from build123d import *

# Parameters (mm, degrees)
SKETCH002_W   = 115
SKETCH002_H   = 101.6
SKETCH002_R   = 3.25
SKETCH002_R_2 = 19.05
SKETCH002_R_3 = 2.1
PAD002_DEPTH  = 6.35
FILLET_R      = 2
SKETCH004_R   = 1.25
SKETCH004_R_2 = 2.75
POCKET_DEPTH  = 6.351


with BuildPart() as part:
    # Sketch002 → Pad002 (new body)
    with BuildSketch(Plane.XZ):
        Rectangle(SKETCH002_W, SKETCH002_H)
        with Locations((19.4, 38.1)):
            Circle(SKETCH002_R, mode=Mode.SUBTRACT)
        with Locations((44.8, 38.1)):
            Circle(SKETCH002_R, mode=Mode.SUBTRACT)
        with Locations((19.4, 12.7)):
            Circle(SKETCH002_R, mode=Mode.SUBTRACT)
        with Locations((44.8, 12.7)):
            Circle(SKETCH002_R, mode=Mode.SUBTRACT)
        with Locations((19.4, -12.7)):
            Circle(SKETCH002_R, mode=Mode.SUBTRACT)
        with Locations((44.8, -12.7)):
            Circle(SKETCH002_R, mode=Mode.SUBTRACT)
        with Locations((19.4, -38.1)):
            Circle(SKETCH002_R, mode=Mode.SUBTRACT)
        with Locations((44.8, -38.1)):
            Circle(SKETCH002_R, mode=Mode.SUBTRACT)
        with Locations((-23.3, -15.1)):
            Circle(SKETCH002_R_2, mode=Mode.SUBTRACT)
        with Locations((-46.85, 8.45)):
            Circle(SKETCH002_R_3, mode=Mode.SUBTRACT)
        with Locations((0.25, 8.45)):
            Circle(SKETCH002_R_3, mode=Mode.SUBTRACT)
        with Locations((-46.85, -38.65)):
            Circle(SKETCH002_R_3, mode=Mode.SUBTRACT)
        with Locations((0.25, -38.65)):
            Circle(SKETCH002_R_3, mode=Mode.SUBTRACT)
    extrude(amount=PAD002_DEPTH)

    # Fillet
    fillet_edges = [part.edges().sort_by_distance(p)[0] for p in [
        (57.5, -3.175, 50.8),
        (57.5, -3.175, -50.8),
        (-57.5, -3.175, -50.8),
        (-57.5, -3.175, 50.8),
    ]]
    fillet(fillet_edges, radius=FILLET_R)

    # Sketch004 (on Face2 of Fillet) → Pocket (cut, through all)
    with BuildSketch(Plane(origin=(0, 0, 0), x_dir=(1, 0, 0), z_dir=(0, 1, 0))):
        with Locations((-14.5, -32.1)):
            Circle(SKETCH004_R)
        with Locations((-14.5, -44.1)):
            Circle(SKETCH004_R)
        with Locations((0.25, -38.1)):
            Circle(SKETCH004_R_2)
    extrude(amount=-POCKET_DEPTH, mode=Mode.SUBTRACT)


solid = part.part
Work out the finished part from the listing and answer in its coordinate system (mm). Give positions to 0.01 mm unless a question says otherwise; leave off trailing zeros. Order: outer loops, then holes, each group sorted by start corner. A loop starts at its lowest first (then second) coordinate and runs counter-clockwise, first axis right, second up. Notation, with made-up numbers: M -29,-5 L -18,-5 A14 cw -18,2 Z; hole C 15.5,22.5 d2. An arc over 180 degrees is marked long. Return JSON: item names as keys, results as strings.
Q1. The mould has two halves that part along Z. Classify faces 1 (the face through (-57.5, -3, -1)), 2 (the face through (47.802, -3.131, 36.855)), 3 (the face through (46.55, -3.13, -35.36)), 4 (the face through (-1, -3, 50.8)): pulls with the +Z half, pulls with the -Z half, needs draft (parallel to the pull), parting line crosses it, or undercut.
Answer below:
{"face 1": "needs draft", "face 2": "undercut", "face 3": "undercut", "face 4": "pulls with the +Z half"}
Q2. Find section B-B, the plane y = -5.25. State how many separate pieces and enclosed holes the cut face has, and give its area (3 significant figures).
Answer below:
{"separate pieces": "1", "enclosed holes": "16", "area": "10,200 mm^2"}
Q3. Find the intervals of material crossed by line 1 along Z through (x, y) = (21.5, -3.75); line 2 along Z through (x, y) = (1, -1.5); line 3 along X through (y, z) = (-4.75, 7), in increasing order. Write a range as [from, to].
Answer below:
{"line 1": "z = [-50.8, -40.58], [-35.62, -15.18], [-10.22, 10.22], [15.18, 35.62], [40.58, 50.8]", "line 2": "z = [-50.8, -40.61], [-36.69, 6.49], [10.41, 35.45], [40.75, 50.8]", "line 3": "x = [-57.5, -48.37], [-45.33, -1.27], [1.77, 57.5]"}
Q4. Find section A-A, the plane z = 44.1. Write down the section's boundary in (x, y), and give its area (3 significant figures).
Answer below:
{"outline": "M -57.5,-6.35 L -15.75,-6.35 L -15.75,0 L -57.5,0 Z; M -13.25,-6.35 L 57.5,-6.35 L 57.5,0 L -13.25,0 Z", "area": "714 mm^2"}
Q5. Find section D-D, the plane x = 44. Write down the section's boundary in (y, z), and give its area (3 significant figures).
Answer below:
{"outline": "M -6.35,-50.8 L 0,-50.8 L 0,-41.25 L -6.35,-41.25 Z; M -6.35,-34.95 L 0,-34.95 L 0,-15.85 L -6.35,-15.85 Z; M -6.35,-9.55 L 0,-9.55 L 0,9.55 L -6.35,9.55 Z; M -6.35,15.85 L 0,15.85 L 0,34.95 L -6.35,34.95 Z; M -6.35,41.25 L 0,41.25 L 0,50.8 L -6.35,50.8 Z", "area": "485 mm^2"}
Q6. Find section C-C, the plane x = -46.85. Write down the section's boundary in (y, z).
Answer below:
{"outline": "M -6.35,-50.8 L 0,-50.8 L 0,-40.75 L -6.35,-40.75 Z; M -6.35,-36.55 L 0,-36.55 L 0,6.35 L -6.35,6.35 Z; M -6.35,10.55 L 0,10.55 L 0,50.8 L -6.35,50.8 Z"}
